from build123d import *

# Parameters (mm, degrees)
F0_W     = 50.8
F0_H     = 76
F0_R     = 1.5
F1_DEPTH = 12.6
F2_R     = 1.5
F3_DEPTH = 10
F4_DEPTH = 50.8
F5_DEPTH = 12
F6_R     = 1.5
F7_DEPTH = 10


with BuildPart() as f1:
    # F0 (on Top) → F1 (new body)
    with BuildSketch(Plane.XY):
        Rectangle(F0_W, F0_H)
        with Locations((-12.5, -25)):
            Circle(F0_R, mode=Mode.SUBTRACT)
        with Locations((12.5, -25)):
            Circle(F0_R, mode=Mode.SUBTRACT)
        with Locations((-12.5, 0)):
            Circle(F0_R, mode=Mode.SUBTRACT)
        Circle(F0_R, mode=Mode.SUBTRACT)
        with Locations((-12.5, 25)):
            Circle(F0_R, mode=Mode.SUBTRACT)
        with Locations((12.5, 0)):
            Circle(F0_R, mode=Mode.SUBTRACT)
        with Locations((12.5, 25)):
            Circle(F0_R, mode=Mode.SUBTRACT)
    extrude(amount=F1_DEPTH)

    # F2 (on face) → F3 (cut)
    with BuildSketch(Plane(origin=(-25.4, 0, 0), x_dir=(0, -1, 0), z_dir=(-1, 0, 0))):
        with Locations((-12.5, 6.3)):
            Circle(F2_R)
        with Locations((12.5, 6.3)):
            Circle(F2_R)
    extrude(amount=-F3_DEPTH, mode=Mode.SUBTRACT)

    # F2 (on face) → F4 (cut)
    with BuildSketch(Plane(origin=(-25.4, 0, 0), x_dir=(0, -1, 0), z_dir=(-1, 0, 0))):
        Polygon((6.3, 12.6), (0, 12.6), (-6.3, 12.6), (0, 6.3), align=None)
    extrude(amount=-F4_DEPTH, mode=Mode.SUBTRACT)

    # F0 (on Top) → F5 (cut)
    with BuildSketch(Plane.XY):
        with Locations((12.5, 0)):
            Circle(F0_R)
        Circle(F0_R)
        with Locations((-12.5, 0)):
            Circle(F0_R)
    extrude(amount=F5_DEPTH, mode=Mode.SUBTRACT)

    # F6 (on face) → F7 (cut)
    with BuildSketch(Plane(origin=(0, 38, 0), x_dir=(-1, 0, 0), z_dir=(0, 1, 0))):
        with Locations((0, 6.3)):
            Circle(F6_R)
    extrude(amount=-F7_DEPTH, mode=Mode.SUBTRACT)


solid = f1.part
Source: CAD feature listing. Evaluate the final solid. Frame: model axes, mm. A direction names the side the tool comes from. Coordinates: 2 decimals unless noted, no trailing zeros. Loops run counter-clockwise (first coordinate to the right, second up) from the corner with the lowest first, then second, coordinate; pieces in that order, holes last. Notation, with made-up numbers: M 61.5,21 L 107.5,21 A15 ccw 107.5,25 Z; hole C 42,53.5 d2. An arc over 180 degrees is marked long. Answer in a Markdown table with one row per item.
Q1. Draft query along Z for faces 4 (the cylindrical face through (-20.47, 12.695, 7.787)), 5 (the cylindrical face through (-12.695, -23.513, 6.212)), 6 (the flat face through (-0.4, 3.2, 9.5)). Return one class per face: pulls with the +Z half, pulls with the -Z half, needs draft (parallel to the pull), parting line crosses it, or undercut.
Answers below:
| item | result |
|---|---|
| face 4 | undercut |
| face 5 | needs draft |
| face 6 | pulls with the +Z half |
Q2. First-contact query: pin 1 (2.5 mm diameter, centred on y = 12.5, z = 6.3, fed in from -X). Flat tip, straight axial feed; report the tip coordinate or a pass-through.
Answers below:
| item | result |
|---|---|
| pin 1 | stops at x = -15.4 |
Q3. Section B-B on x = 0. Return the cut outline in (y, z).
Answers below:
| item | result |
|---|---|
| outline | M -38,0 L -1.5,0 L -1.5,7.8 L -6.3,12.6 L -38,12.6 Z; M 1.5,0 L 38,0 L 38,4.8 L 28,4.8 L 28,7.8 L 38,7.8 L 38,12.6 L 6.3,12.6 L 1.5,7.8 Z |
Q4. Set-up query: faces 1 (the flat face through (-15.4, 13, 6)), 2 (the flat face through (0, 28, 6)), 3 (the flat face through (-0.4, -3.1, 9.4)). Return all of +Z, -Z, +X, -X, +Y, -Y with unobstructed straight access to the full face (end or side cutting, diameter ignored); none if empty.
Answers below:
| item | result |
|---|---|
| face 1 | -X |
| face 2 | +Y |
| face 3 | +Z, +X, -X |
Q5. Ray query, probe 1 along Y at (x, z) = (12.5, 3.25); probe 2 along X at (y, z) = (0, 4.25); probe 3 along Z at (x, y) = (0, 31.25). Return the intervals inside material, ascending. Write a range as from..to.
Answers below:
| item | result |
|---|---|
| probe 1 | y = -38..-26.5, -23.5..-1.5, 1.5..23.5, 26.5..38 |
| probe 2 | x = -25.4..-14, -11..-1.5, 1.5..11, 14..25.4 |
| probe 3 | z = 0..4.8, 7.8..12.6 |
Q6. Section D-D on x = 12.5. Return the cut outline in (y, z), plus the area to 3 significant figures.
Answers below:
| item | result |
|---|---|
| outline | M -38,0 L -26.5,0 L -26.5,12.6 L -38,12.6 Z; M -23.5,0 L -1.5,0 L -1.5,7.8 L -6.3,12.6 L -23.5,12.6 Z; M 1.5,0 L 23.5,0 L 23.5,12.6 L 6.3,12.6 L 1.5,7.8 Z; M 26.5,0 L 38,0 L 38,12.6 L 26.5,12.6 Z |
| area | 821 mm^2 |
Q7. Section A-A on z = 11.25. Return the cut outline in (x, y).
Answers below:
| item | result |
|---|---|
| outline | M -25.4,-38 L 25.4,-38 L 25.4,-4.95 L -25.4,-4.95 Z; M -25.4,4.95 L 25.4,4.95 L 25.4,38 L -25.4,38 Z; hole C -12.5,-25 d3; hole C -12.5,25 d3; hole C 12.5,-25 d3; hole C 12.5,25 d3 |
Q8. Section C-C on x = -21. Return the cut outline in (y, z), plus the area to 3 significant figures.
Answers below:
| item | result |
|---|---|
| outline | M -38,0 L 38,0 L 38,12.6 L 6.3,12.6 L 0,6.3 L -6.3,12.6 L -38,12.6 Z; hole C -12.5,6.3 d3; hole C 12.5,6.3 d3 |
| area | 904 mm^2 |
